Check sheet for the modelled part. Datum: model origin and axes. Units: mm. Face numbers are marked on the shaded views. Coordinates: 2 decimals unless noted, no trailing zeros. Loops run counter-clockwise (first coordinate to the right, second up) from the corner with the lowest first, then second, coordinate; pieces in that order, holes last. Notation, with made-up numbers: (-29, 20) -> (-6, 20) arc R20 ccw to (-6, 49) -> close; hole circle Ø2 at (63, -21). An arc over 180 degrees is marked (long way). Use one line per item in the form item = value.
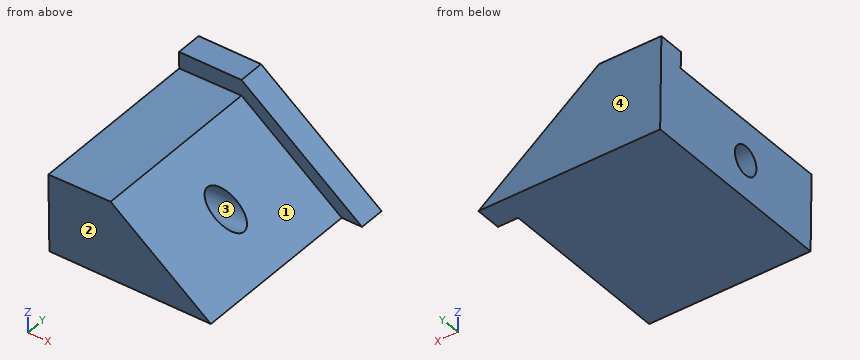
from build123d import *

# Parameters (mm, degrees)
F1_DEPTH = 76.2
F3_DEPTH = 66.294
F4_R     = 5.442809
F5_DEPTH = 87.884


with BuildPart() as f1:
    # F0 (on Front) → F1 (new body)
    with BuildSketch(Plane.XZ):
        Polygon((-34.636363, 35.213638), (-34.174547, 0), (34.405455, 0), (-11.083637, 35.213638), align=None)
    extrude(amount=F1_DEPTH)

    # F2 (on face) → F3 (cut)
    with BuildSketch(Plane.XZ.offset(76.2)):
        Polygon((-11.083637, 29.291008), (26.754583, 0), (34.405455, 0), (-11.083637, 35.213638), (-34.636363, 35.213638), (-34.554653, 28.983193), align=None)
    extrude(amount=-F3_DEPTH, mode=Mode.SUBTRACT)

    # F4 (on face) → F5 (cut)
    with BuildSketch(Plane(origin=(-34.16867, 0, -0.448112), x_dir=(0, -1, 0), z_dir=(-0.999914, 0, -0.013114))):
        with Locations((43.053, 14.650282)):
            Circle(F4_R)
    extrude(amount=-F5_DEPTH, mode=Mode.SUBTRACT)


solid = f1.part
(1) Mould release check, pull along Y, two halves, no side actions. Record for the marked faces 1, 2, 3 and 4: +Y half, -Y half, draft (parallel to the pull), parting line (faces both ways), or undercut.
Established:
face_1 = draft
face_2 = -Y half
face_3 = undercut
face_4 = +Y half
(2) Scan lines: line 1 along Y through (x, z) = (-4, 26); line 2 along Z through (x, y) = (-19, -39); line 3 along Y through (x, z) = (-10, 16). Record each from-to range of solid material in increasing order.
Established:
line_1 = -9.91 to 0
line_2 = 0 to 10.77, 18.04 to 29.19
line_3 = -76.2 to -48.29, -37.82 to 0
(3) Section check A-A, the plane x = 23.5. Record the boundary of the cut face in (y, z), plus the area to 3 significant figures.
Established:
outline = (-76.2, 0) -> (0, 0) -> (0, 8.44) -> (-9.91, 8.44) -> (-9.91, 2.52) -> (-76.2, 2.52) -> close
area = 251 mm²
(4) Section check D-D, the plane y = -9. Record the boundary of the cut face in (x, z).
Established:
outline = (-34.64, 35.21) -> (-34.17, 0) -> (34.41, 0) -> (-11.08, 35.21) -> close
(5) Section check C-C, the plane z = 22. Record the boundary of the cut face in (x, y), plus the area to 4 significant figures.
Established:
outline = (-34.46, -76.2) -> (-1.67, -76.2) -> (-1.67, -9.91) -> (5.99, -9.91) -> (5.99, 0) -> (-34.46, 0) -> close
area = 2,575 mm²
(6) Go/stop test with flat-tipped pins: P1, Ø2, axis at y = -66.5, z = 20.5, coming from the +X side; P2, Ø6, axis at y = -26.5, z = 31.5, coming from the -X side; P3, Ø1, axis at y = -16.5, z = 28, coming from the +X side. Record where each tip stops, or that it passes through.
Established:
P1 = 1.56
P2 = -34.55
P3 = -8.77
(7) Section check B-B, the plane y = -34.5. Record the boundary of the cut face in (x, z).
Established:
outline = (-34.55, 28.98) -> (-34.17, 0) -> (26.75, 0) -> (-11.08, 29.29) -> close
